```python
from build123d import *

# Parameters (mm, degrees)
F0_R     = 6
F1_DEPTH = 20
F2_R     = 6
F3_R     = 3.25
F4_DEPTH = 18
F5_R     = 3


with BuildPart() as f1:
    # F0 (on Top) → F1 (new body)
    with BuildSketch(Plane.XY):
        Circle(F0_R)
    extrude(amount=F1_DEPTH)

    # F2
    f2_edges = [f1.edges().sort_by_distance(p)[0] for p in [
        (-6, 0, 20),
    ]]
    fillet(f2_edges, radius=F2_R)

    # F3 (on face) → F4 (cut)
    with BuildSketch(Plane(origin=(0, 0, 0), x_dir=(1, 0, 0), z_dir=(0, 0, -1))):
        Circle(F3_R)
    extrude(amount=-F4_DEPTH, mode=Mode.SUBTRACT)

    # F5
    f5_edges = [f1.edges().sort_by_distance(p)[0] for p in [
        (-3.25, 0, 18),
    ]]
    fillet(f5_edges, radius=F5_R)


solid = f1.part
```
Check sheet for the modelled part. Datum: model origin and axes. Units: mm. A direction names the side the tool comes from. Coordinates: 2 decimals unless noted, no trailing zeros. Write each loop counter-clockwise with the first axis right and the second up, starting at its lowest first coordinate (ties: lowest second). Pieces come first, ordered by that corner, then holes. Notation, with made-up numbers: M -3.75,-32 L 36.25,-32 A15 ccw 36.25,-27 Z; hole C 3,-6 d10. An arc over 180 degrees is marked long. Write item = value, one per line. Start each with the question number.
1. Sectioned sample at A-A (z = 13). Record the cut outline in (x, y).
2. Sectioned sample at B-B (x = -4.75). Record the cut outline in (y, z), then the cut area to 3 significant figures.
3. Go/stop test with flat-tipped pins: pin 1 (1.5 mm diameter, centred on y = -0.5, z = 16, fed in from +X); pin 2 (1 mm diameter, centred on x = 1, z = 14.5, fed in from +Y); pin 3 (1 mm diameter, centred on x = -4, z = 13.5, fed in from +Y). Record where each tip stops, or that it passes through.
4. Sectioned sample at C-C (z = 18.5). Record the cut outline in (x, y).
5. Tool access check on faces 1 (the cylindrical face through (-2.579, 1.978, 7.395)), 2 (the cylindrical face through (-6, 0, 7)). Record the directions out of +Z, -Z, +X, -X, +Y, -Y that give a thin tool (end or side, any length) a straight path to the whole face; none if there is none.
6. Thickness scan on probe 1 along Y at (x, z) = (0, 11.75); probe 2 along X at (y, z) = (-3, 11); probe 3 along Y at (x, z) = (2, 1). Record the ranges inside material, lowest first.
The answers:
q1.outline = C 0,0 d12; hole C 0,0 d6.5
q2.outline = M -3.67,0 L 3.67,0 L 3.67,14 A3.67 ccw -3.67,14 Z
q2.area = 124 mm²
q3.pin_1 = 5.85
q3.pin_2 = 5.97
q3.pin_3 = 4.87
q4.outline = C 0,0 d7.94
q5.face_1 = -Z
q5.face_2 = +Z, -Z
q6.probe_1 = -6 to -3.25, 3.25 to 6
q6.probe_2 = -5.2 to -1.25, 1.25 to 5.2
q6.probe_3 = -5.66 to -2.56, 2.56 to 5.66
